Verification items for the finished model (mm, model axes). A direction names the side the tool comes from. Coordinates: 2 decimals unless noted, no trailing zeros. Write each loop counter-clockwise with the first axis right and the second up, starting at its lowest first coordinate (ties: lowest second). Pieces come first, ordered by that corner, then holes. Notation, with made-up numbers: (-14.75, 85.5) -> (-1.75, 85.5) arc R29 ccw to (-1.75, 122.5) -> close; hole circle Ø9 at (12.5, 13). An arc over 180 degrees is marked (long way). Answer in a Markdown table with one row per item.
Autodesk Inventor part; units mm, degrees
ref_plane "YZ Plane" through (0, 0, 0) normal (1, 0, 0) x (0, 1, 0)
ref_plane "XZ Plane" through (0, 0, 0) normal (0, 1, 0) x (-1, 0, 0)
ref_plane "XY Plane" through (0, 0, 0) normal (0, 0, 1) x (1, 0, 0)
sketch "Sketch1" plane through (0, 0, 0) normal (0, 1, 0) x (-1, 0, 0)
  line L0 (0, 0) -> (260.0718, 0)
  line L1 (260.0718, 0) -> (260.0718, -6.35)
  line L2 (260.0718, -6.35) -> (0, -6.35)
  line L3 (0, -6.35) -> (0, 0)
  dimension "d0" = 260.0718
  dimension "d1" = 6.35
extrude "Extrusion1" add sketch "Sketch1" along normal blind 6.35
sketch "Sketch2" plane through (-260.0718, 0, -6.35) normal (-1, 0, 0) x (0, 0, 1)
  line L0 (6.35, 6.35) -> (0, 6.35)
  line L1 (6.35, 0) -> (6.35, 6.35)
  circle A0 centre (3.175, 3.175) radius 3.175
  dimension "d4" = 3.175
  dimension "d5" = 3.175
  dimension "d6" = 6.35
extrude "Extrusion2" add sketch "Sketch2" along normal blind 6.35 contours A0
sketch "Sketch3" plane through (0, 0, 0) normal (1, 0, 0) x (0, 0, -1)
  line L0 (0, 6.35) -> (6.35, 6.35)
  line L1 (6.35, 0) -> (6.35, 6.35)
  circle A0 centre (3.175, 3.175) radius 3.175
  point P0 (0, 0)
  dimension "d9" = 3.175
  dimension "d10" = 3.175
  dimension "d11" = 6.35
extrude "Extrusion3" add sketch "Sketch3" along normal blind 6.35 contours A0
sketch "Sketch4" plane through (6.35, 3.175, -3.175) normal (1, 0, 0) x (0, 0, -1)
  circle A0 centre (0, 0) radius 6.35
  point P0 (-3.175, -3.175)
  dimension "d14" = 12.7
extrude "Extrusion4" add sketch "Sketch4" along normal blind 1.5875
equation "\"d0\" = -6 * SpWall + IBDia"
equation "\"d1\" = AxelDia"
equation "\"d2\" = AxelDia"
equation "\"d6\" = AxelDia"
equation "\"d7\" = 2 * SpWall"
equation "\"d11\" = AxelDia"
equation "\"d12\" = 2 * SpWall"
equation "\"d15\" = Wall"
properties part number "MotorMntPart"
1. Tool access check on faces 4 (the flat face through (-128, 0, -3)), 5 (the flat face through (-128, 3, 0)), 6 (the cylindrical face through (-263.2, 4.39, -0.24)). Record the directions out of +Z, -Z, +X, -X, +Y, -Y that give a thin tool (end or side, any length) a straight path to the whole face; none if there is none.
Geometry says:
| item | result |
|---|---|
| face 4 | +Z, -Z, -X, -Y |
| face 5 | +Z, -X, +Y, -Y |
| face 6 | -X |
2. Mould release check, pull along X, two halves, no side actions. Record for faces 1 (the flat face through (-132, 3, -6.35)), 2 (the flat face through (7.938, 3, -3)), 3 (the cylindrical face through (3.131, 6.274, -2.487)): released by +X, released by -X, zero draft, split by the parting line, or undercut.
Geometry says:
| item | result |
|---|---|
| face 1 | zero draft |
| face 2 | released by +X |
| face 3 | undercut |
3. Depth check by flat-ended pin: P1, Ø6, axis at x = -53.5, z = 2, coming from the +Y side; P2, Ø2, axis at x = -155, z = -2, coming from the -Y side; P3, Ø3, axis at x = -144.5, y = 2.5, coming from the -Z side. Enter the tip coordinate at first touch or a pass-through.
Geometry says:
| item | result |
|---|---|
| P1 | y = 6.35 |
| P2 | y = 0 |
| P3 | z = -6.35 |
4. Section check A-A, the plane x = -189.5. Record the boundary of the cut face in (y, z), plus the area to 3 significant figures.
Geometry says:
| item | result |
|---|---|
| outline | (0, -6.35) -> (6.35, -6.35) -> (6.35, 0) -> (0, 0) -> close |
| area | 40.3 mm^2 |
5. Thickness scan on line 1 (X direction, y = 1, z = -6.25); line 2 (Y direction, x = -165.5, z = -3.5); line 3 (Z direction, x = -20.5, y = 4). Record the ranges inside material, lowest first. Write a range as from..to.
Geometry says:
| item | result |
|---|---|
| line 1 | -260.07..0, 6.35..7.94 |
| line 2 | 0..6.35 |
| line 3 | -6.35..0 |
